Geometry check sheet. Reference: the model listing, model coordinates, mm. Round coordinates to 2 decimals unless told otherwise and drop trailing zeros. Order: outer loops, then holes, each group sorted by start corner. A loop starts at its lowest first (then second) coordinate and runs counter-clockwise, first axis right, second up.
(1) Release check for a two-part mould opening along X. For faces 1 (the face through (23.19, 49.94, -10.88)), 2 (the face through (16, 58.687, -11)), 3 (the face through (2.886, -7, -11)) record: +X half, -X half, draft (parallel to the pull), parting line (faces both ways), or undercut.
(2) Material ranges on line 1 along Y through (x, z) = (23.5, -18); line 2 along Y through (x, z) = (21.5, -10), recorded low to high.
(3) Sectioned sample at B-B (z = -2.75). Record the boundary of the cut face in (x, y).
(4) Sectioned sample at A-A (x = 10.25). Record the boundary of the cut face in (y, z).
(5) Go/stop test with flat-tipped pins: pin 1 (5 mm diameter, centred on x = 24.5, y = -39.5, fed in from +Z); pin 2 (3.5 mm diameter, centred on x = 8.84, y = 47.01, fed in from -Z). Record where each tip stops, or that it passes through.
(6) Sectioned sample at C-C (x = 23.5). Record the boundary of the cut face in (y, z), plus the area to 3 significant figures.
from build123d import *

# Parameters (mm, degrees)
ESBO_O1_W             = 26.9
ESBO_O1_H             = 129.35
FLANGE_BASE1_DEPTH    = 21.45
ESBO_O7_R             = 3
CORTE_EXTRUS_O1_DEPTH = 21.45


# Sheet-metal steps are written as plain solids
with BuildPart() as part:
    # Esboço1 → Flange-base1 (new body)
    with BuildSketch(Plane.XY):
        with Locations((16.336467182, -5.988425926)):
            Rectangle(ESBO_O1_W, ESBO_O1_H)
    extrude(amount=-FLANGE_BASE1_DEPTH)

    # Esboço7 → Corte-extrusão1 (cut)
    with BuildSketch(Plane(origin=(0, 0, -21.45), x_dir=(-1, 0, 0), z_dir=(0, 0, -1))):
        with Locations(Location((-23.836467182, 47.011574074, 0), (0, 0, 180))):
            Circle(ESBO_O7_R)
        with Locations(Location((-8.836467182, 47.011574074, 0), (0, 0, 180))):
            Circle(ESBO_O7_R)
        with Locations(Location((-23.836467182, -58.988425926, 0), (0, 0, 180))):
            Circle(ESBO_O7_R)
        with Locations(Location((-8.836467182, -58.988425926, 0), (0, 0, 180))):
            Circle(ESBO_O7_R)
    extrude(amount=-CORTE_EXTRUS_O1_DEPTH, mode=Mode.SUBTRACT)


solid = part.part
Answer below:
1. face 1: undercut
1. face 2: draft
1. face 3: -X half
2. line 1: y = -70.66 to -61.97, -56.01 to 44.03, 49.99 to 58.69
2. line 2: y = -70.66 to -60.87, -57.11 to 45.13, 48.89 to 58.69
3. outline: (2.89, -70.66) - (29.79, -70.66) - (29.79, 58.69) - (2.89, 58.69) - close; hole circle Ø6 at (8.84, -58.99); hole circle Ø6 at (8.84, 47.01); hole circle Ø6 at (23.84, -58.99); hole circle Ø6 at (23.84, 47.01)
4. outline: (-70.66, -21.45) - (-61.63, -21.45) - (-61.63, 0) - (-70.66, 0) - close; (-56.34, -21.45) - (44.37, -21.45) - (44.37, 0) - (-56.34, 0) - close; (49.66, -21.45) - (58.69, -21.45) - (58.69, 0) - (49.66, 0) - close
5. pin 1: stops at z = 0
5. pin 2: passes through
6. outline: (-70.66, -21.45) - (-61.97, -21.45) - (-61.97, 0) - (-70.66, 0) - close; (-56.01, -21.45) - (44.03, -21.45) - (44.03, 0) - (-56.01, 0) - close; (49.99, -21.45) - (58.69, -21.45) - (58.69, 0) - (49.99, 0) - close
6. area: 2,520 mm2
